```python
from build123d import *

# Parameters (mm, degrees)
F0_W     = 37.5
F0_H     = 52.5
F1_DEPTH = 1
F0_H_2   = 1
F2_DEPTH = 18.5
F4_DEPTH = 60
F5_DEPTH = 20
F6_R     = 2
F7_R     = 2


with BuildPart() as f1:
    # F0 (on Top) → F1 (new body)
    with BuildSketch(Plane.XY):
        Rectangle(F0_W, F0_H)
    extrude(amount=F1_DEPTH)

    # F0 (on Top) → F2 (join)
    with BuildSketch(Plane.XY):
        with Locations((0, 26.75)):
            Rectangle(F0_W, F0_H_2)
        with Locations((0, -26.75)):
            Rectangle(F0_W, F0_H_2)
    extrude(amount=F2_DEPTH)

    # F3 (on face) → F4 (cut)
    with BuildSketch(Plane.XZ.offset(27.25)):
        with BuildLine():
            ThreePointArc((4, 15), (3.8535533906, 15.3535533906), (3.5, 15.5))
            Line((3.5, 15.5), (-3.5, 15.5))
            ThreePointArc((-3.5, 15.5), (-3.8535533906, 15.3535533906), (-4, 15))
            Line((-4, 15), (-4, 13.5))
            ThreePointArc((-4, 13.5), (-3.8535533906, 13.1464466094), (-3.5, 13))
            Line((-3.5, 13), (3.5, 13))
            ThreePointArc((3.5, 13), (3.8535533906, 13.1464466094), (4, 13.5))
            Line((4, 13.5), (4, 15))
        make_face()
    extrude(amount=-F4_DEPTH, mode=Mode.SUBTRACT)

    # F0 (on Top) → F5 (join)
    with BuildSketch(Plane.XY):
        Polygon((-18.75, -26.25), (-18.75, 26.25), (-18.75, 27.25), (-19.75, 27.25), (-19.75, -27.25), (-18.75, -27.25), align=None)
        Polygon((18.75, 27.25), (18.75, 26.25), (18.75, -26.25), (18.75, -27.25), (19.75, -27.25), (19.75, 27.25), align=None)
    extrude(amount=F5_DEPTH)

    # F6
    f6_edges = [f1.edges().sort_by_distance(p)[0] for p in [
        (19.75, -27.25, 10),
        (-19.75, -27.25, 10),
        (19.75, 27.25, 10),
        (-19.75, 27.25, 10),
    ]]
    fillet(f6_edges, radius=F6_R)

    # F7
    f7_edges = [f1.edges().sort_by_distance(p)[0] for p in [
        (-19.75, 0, 0),
        (-19.164214, -26.664214, 0),
        (0, -27.25, 0),
        (19.164214, -26.664214, 0),
        (19.75, 0, 0),
        (19.164214, 26.664214, 0),
        (0, 27.25, 0),
        (-19.164214, 26.664214, 0),
    ]]
    fillet(f7_edges, radius=F7_R)


solid = f1.part
```
Input: part model. Units: mm. Frame: model coordinates. A direction names the side the tool comes from. Give positions to 0.01 mm unless a question says otherwise; leave off trailing zeros. Order: outer loops, then holes, each group sorted by start corner. A loop starts at its lowest first (then second) coordinate and runs counter-clockwise, first axis right, second up. Notation, with made-up numbers: (31, 75) - (66, 75) arc R16 ccw to (66, 93) - close; hole circle Ø6 at (15.5, 69). An arc over 180 degrees is marked (long way). Use a Markdown table: item, result.
(1) Pin query (flat end, axial travel): pin 1 (0.8 mm diameter, centred on y = 26.5, z = 14.5, fed in from -X); pin 2 (0.5 mm diameter, centred on x = -7, y = -26.5, fed in from +Z); pin 3 (1.5 mm diameter, centred on x = -8, y = -21.5, fed in from +Z). Return the tip coordinate at first contact, or that it passes through.
Computed values:
| item | result |
|---|---|
| pin 1 | stops at x = -19.56 |
| pin 2 | stops at z = 18.5 |
| pin 3 | stops at z = 1 |
(2) Line query: line 1 (Y direction, x = -12, z = 4.25); line 2 (X direction, y = -3, z = 19.25); line 3 (Z direction, x = 16, y = 10.5). Output: solid intervals per line, ascending. Write a range as from..to.
Computed values:
| item | result |
|---|---|
| line 1 | y = -27.25..-26.25, 26.25..27.25 |
| line 2 | x = -19.75..-18.75, 18.75..19.75 |
| line 3 | z = 0..1 |
(3) Section query D-D (y = -6.5). Output: boundary loops of the cut face in (x, z), then the cut area to 3 significant figures.
Computed values:
| item | result |
|---|---|
| outline | (-19.75, 2) arc R2 ccw to (-17.75, 0) - (17.75, 0) arc R2 ccw to (19.75, 2) - (19.75, 20) - (18.75, 20) - (18.75, 1) - (-18.75, 1) - (-18.75, 20) - (-19.75, 20) - close |
| area | 75.8 mm2 |
(4) Section query C-C (z = 9.5). Output: boundary loops of the cut face in (x, y).
Computed values:
| item | result |
|---|---|
| outline | (-19.75, -25.25) arc R2 ccw to (-17.75, -27.25) - (17.75, -27.25) arc R2 ccw to (19.75, -25.25) - (19.75, 25.25) arc R2 ccw to (17.75, 27.25) - (-17.75, 27.25) arc R2 ccw to (-19.75, 25.25) - close; hole (-18.75, -26.25) - (18.75, -26.25) - (18.75, 26.25) - (-18.75, 26.25) - close |
(5) Access query for faces 1 (the cylindrical face through (-19.15, -0.35, 0.57)), 2 (the flat face through (0, -26.25, 10)). Directions: +Z, -Z, +X, -X, +Y, -Y. A direction counts if a zero-diameter tool reaches every point of the face in a straight line with its end or side. Return the directions, or none.
Computed values:
| item | result |
|---|---|
| face 1 | -Z, -X, +Y, -Y |
| face 2 | +Z |
(6) Section query B-B (x = -11). Output: boundary loops of the cut face in (y, z), then the cut area to 3 significant figures.
Computed values:
| item | result |
|---|---|
| outline | (-27.25, 2) arc R2 ccw to (-25.25, 0) - (25.25, 0) arc R2 ccw to (27.25, 2) - (27.25, 18.5) - (26.25, 18.5) - (26.25, 1) - (-26.25, 1) - (-26.25, 18.5) - (-27.25, 18.5) - close |
| area | 87.8 mm2 |
(7) Draft query along X for faces 3 (the cylindrical face through (19.15, 26.68, 11.13)), 4 (the flat face through (0, 0, 0)), 5 (the flat face through (0, 26.25, 10)). Return one class per face: released by +X, released by -X, zero draft, split by the parting line, or undercut.
Computed values:
| item | result |
|---|---|
| face 3 | released by +X |
| face 4 | zero draft |
| face 5 | undercut |
(8) Section query A-A (z = 14.25). Output: boundary loops of the cut face in (x, y).
Computed values:
| item | result |
|---|---|
| outline | (-19.75, -25.25) arc R2 ccw to (-17.75, -27.25) - (-4, -27.25) - (-4, -26.25) - (-18.75, -26.25) - (-18.75, 26.25) - (-4, 26.25) - (-4, 27.25) - (-17.75, 27.25) arc R2 ccw to (-19.75, 25.25) - close; (4, -27.25) - (17.75, -27.25) arc R2 ccw to (19.75, -25.25) - (19.75, 25.25) arc R2 ccw to (17.75, 27.25) - (4, 27.25) - (4, 26.25) - (18.75, 26.25) - (18.75, -26.25) - (4, -26.25) - close |
